Check sheet for the modelled part. Datum: model origin and axes. Units: mm. Face numbers are marked on the shaded views. A direction names the side the tool comes from. Give positions to 0.01 mm unless a question says otherwise; leave off trailing zeros. Order: outer loops, then holes, each group sorted by start corner. A loop starts at its lowest first (then second) coordinate and runs counter-clockwise, first axis right, second up. Notation, with made-up numbers: M 87,31.5 L 137,31.5 A17 ccw 137,62.5 Z; hole C 54.5,65.5 d3. An arc over 180 degrees is marked long. Return JSON: item names as keys, results as strings. Group by question number.
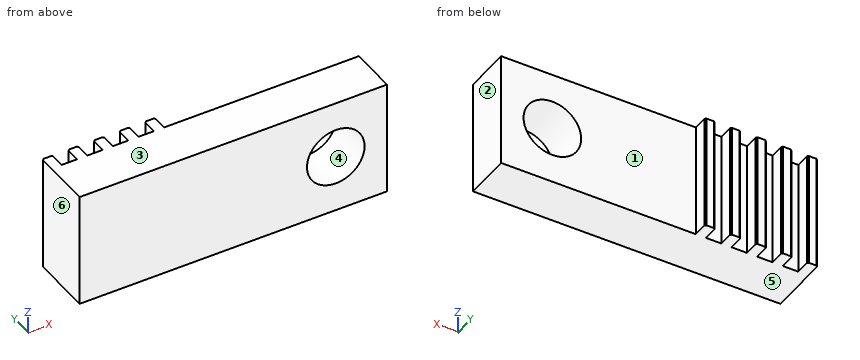
from build123d import *

# Parameters (mm, degrees)
BOSS_EXTRUDE1_DEPTH = 9
CHAMFER1_SIZE       = 0.1
SKETCH2_R           = 2.25
CUT_EXTRUDE1_DEPTH  = 4.65


with BuildPart() as part:
    # Sketch1 → Boss-Extrude1 (new body)
    with BuildSketch(Plane.XY):
        Polygon((28, 3.65), (28, 0), (4, 0), (4, 3.65), (4, 4.85), (4.8, 4.85), (4.8, 3.65), (6, 3.65), (6, 4.85), (6.8, 4.85), (6.8, 3.65), (8, 3.65), (8, 4.85), (8.8, 4.85), (8.8, 3.65), (10, 3.65), (10, 4.85), (10.8, 4.85), (10.8, 3.65), (12, 3.65), (12, 4.85), (12.8, 4.85), (12.8, 3.65), align=None)
    extrude(amount=BOSS_EXTRUDE1_DEPTH)

    # Chamfer1
    chamfer1_edges = [part.edges().sort_by_distance(p)[0] for p in [
        (4, 4.85, 4.5),
        (4.8, 4.85, 4.5),
        (6, 4.85, 4.5),
        (6.8, 4.85, 4.5),
        (8, 4.85, 4.5),
        (8.8, 4.85, 4.5),
        (10, 4.85, 4.5),
        (10.8, 4.85, 4.5),
        (12, 4.85, 4.5),
        (12.8, 4.85, 4.5),
    ]]
    chamfer(chamfer1_edges, length=CHAMFER1_SIZE)

    # Sketch2 → Cut-Extrude1 (cut, through all)
    with BuildSketch(Plane(origin=(0, 3.65, 0), x_dir=(1, 0, 0), z_dir=(0, 1, 0))):
        with Locations((24, -4.5)):
            Circle(SKETCH2_R)
    extrude(amount=-CUT_EXTRUDE1_DEPTH, mode=Mode.SUBTRACT)


solid = part.part
1) Tool access check on the marked faces 1 and 2. Record the directions out of +Z, -Z, +X, -X, +Y, -Y that give a thin tool (end or side, any length) a straight path to the whole face; none if there is none.
2) Sectioned sample at C-C on y = 0.5. Record the boundary of the cut face in (x, z).
3) Sectioned sample at A-A on x = 24. Record the boundary of the cut face in (y, z), then the cut area to 3 significant figures.
4) Sectioned sample at B-B on y = 4.1. Record the boundary of the cut face in (x, z), then the cut area to 3 significant figures.
5) Release check for a two-part mould opening along Z. For the marked faces 3, 4, 5 and 6 record: released by +Z, released by -Z, zero draft, split by the parting line, or undercut.
6) Material ranges on line 1 along X through (y, z) = (2.7, 4.5); line 2 along Z through (x, y) = (24, 2.75); line 3 along Y through (x, z) = (22.5, 1.5), recorded low to high.
7) Depth check by flat-ended pin: P1, Ø0.6, axis at y = 4, z = 3.5, coming from the +X side. Enter the tip coordinate at first touch or a pass-through.
Reply:
{
 "1": {"face 1": "+Z, -Z, +X, +Y", "face 2": "+Z, -Z, +X, +Y, -Y"},
 "2": {"outline": "M 4,0 L 28,0 L 28,9 L 4,9 Z; hole C 24,4.5 d4.5"},
 "3": {"outline": "M 0,0 L 3.65,0 L 3.65,2.25 L 0,2.25 Z; M 0,6.75 L 3.65,6.75 L 3.65,9 L 0,9 Z", "area": "16.4 mm^2"},
 "4": {"outline": "M 4,0 L 4.8,0 L 4.8,9 L 4,9 Z; M 6,0 L 6.8,0 L 6.8,9 L 6,9 Z; M 8,0 L 8.8,0 L 8.8,9 L 8,9 Z; M 10,0 L 10.8,0 L 10.8,9 L 10,9 Z; M 12,0 L 12.8,0 L 12.8,9 L 12,9 Z", "area": "36.0 mm^2"},
 "5": {"face 3": "released by +Z", "face 4": "undercut", "face 5": "released by -Z", "face 6": "zero draft"},
 "6": {"line 1": "4 to 21.75, 26.25 to 28", "line 2": "0 to 2.25, 6.75 to 9", "line 3": "0 to 3.65"},
 "7": {"P1": "x = 12.8"}
}
